Build history of the part. All positions in model axes, mm. A direction names the side the tool comes from. Round coordinates to 2 decimals unless told otherwise and drop trailing zeros. Order: outer loops, then holes, each group sorted by start corner. A loop starts at its lowest first (then second) coordinate and runs counter-clockwise, first axis right, second up. Notation, with made-up numbers: (61, 52) - (91, 52) arc R20 cw to (91, 60) - close; hole circle Ø10 at (16.25, -35.75). An arc over 180 degrees is marked (long way). Write each question's results on one line, items separated by ' | '. Start each with the question number.
```python
from build123d import *

# Parameters (mm, degrees)
F1_DEPTH    = 41
F2_R        = 4
F3_T1_DEPTH = 51


# Not quite as in the source:
# - a fillet or chamfer that OpenCascade refuses, or shapes differently, is made with other operations: its cross-section is extruded or revolved along the edge and cut away or added


with BuildPart() as f1:
    # F0 (on Front) → F1 (new body)
    with BuildSketch(Plane.XZ):
        Polygon((-42.5, 18.5), (-39, 18.5), (-39, 38.5), (-17.5, 38.5), (-17.5, 21.5), (-3.5, 21.5), (-3.5, -3.5), (0, -3.5), (0, 0), (0, 25), (-14, 25), (-14, 42), (-42.5, 42), align=None)
        Polygon((0, 0), (0, -3.5), (33.5, -3.5), (33.5, -147.2), (13.5, -147.2), (13.5, -150.7), (37, -150.7), (37, 0), align=None)
    extrude(amount=F1_DEPTH)

    # F2
    f2_edges = [f1.edges().sort_by_distance(p)[0] for p in [
        (-42.5, -20.5, 42),
        (-14, -20.5, 42),
        (0, -20.5, 25),
        (0, -20.5, 0),
        (-14, -20.5, 25),
        (37, -20.5, 0),
        (37, -20.5, -150.7),
        (-3.5, -20.5, -3.5),
    ]]
    fillet(f2_edges, radius=F2_R)

    # F3: fillet of radius 2 on 4 edges, made by hand

    # F3_s2 → F3_t1 (cut)
    with BuildSketch(Plane.XZ.offset(-5)):
        with BuildLine():
            ThreePointArc((-40.5, 18.5), (-41.9142135624, 19.0857864376), (-42.5, 20.5))
            Line((-42.5, 20.5), (-42.5, 18.5))
            Line((-42.5, 18.5), (-40.5, 18.5))
        make_face()
        with BuildLine():
            ThreePointArc((15.5, -147.2), (14.0857864376, -147.7857864376), (13.5, -149.2))
            Line((13.5, -149.2), (13.5, -147.2))
            Line((13.5, -147.2), (15.5, -147.2))
        make_face()
        with BuildLine():
            ThreePointArc((13.5, -148.7), (14.0857864376, -150.1142135624), (15.5, -150.7))
            Line((15.5, -150.7), (13.5, -150.7))
            Line((13.5, -150.7), (13.5, -148.7))
        make_face()
        with BuildLine():
            ThreePointArc((-15.5, 21.5), (-16.9142135624, 22.0857864376), (-17.5, 23.5))
            Line((-17.5, 23.5), (-17.5, 21.5))
            Line((-17.5, 21.5), (-15.5, 21.5))
        make_face()
    extrude(amount=F3_T1_DEPTH, mode=Mode.SUBTRACT)


solid = f1.part
```
1. Cut at D-D (x = -8). List the corners of the cut face in (y, z), plus the area to 4 significant figures.
2. 3-axis set-ups, long thin cutter, end or side, ignore diameter. For faces 5 (the face through (0, -20, 12)), 6 (the face through (17, -20, -3.5)), 7 (the face through (-42.5, -20, 29)): which of +Z, -Z, +X, -X, +Y, -Y reach the whole face in a straight line?
3. Cut at C-C (z = -129). List the corners of the cut face in (x, y).
4. Cut at B-B (x = 19.5). List the corners of the cut face in (y, z).
5. Wall check: line 1 (X direction, y = -13, z = 34); line 2 (Z direction, x = 25, y = -9.5); line 3 (Z direction, x = -8.5, y = -23.5). Give the ranges that are in metal, low to high. Write a range as from..to.
6. Flat gauge pins, fed straight in: pin 1 Ø1.5 at (y, z) = (-11.5, -0.5) entering from +X; pin 2 Ø6.5 at (x, y) = (-8, -24.5) entering from +Z; pin 3 Ø11 at (x, y) = (-28, -15.5) entering from -Z; pin 4 Ø23 at (y, z) = (-27, 10) entering from -X. Where does each tip first touch, or does it go through?
7. Mould opens along Z. For faces 1 (the face through (-3, -41, 3)), 2 (the face through (25, -20, -147.2)), 3 (the face through (-7, -20, 25)), 4 (the face through (-2.359, -20.787, -2.297)) say: pulls with the +Z half, pulls with the -Z half, needs draft (parallel to the pull), parting line crosses it, or undercut.
A:
1) outline: (-41, 21.5) - (0, 21.5) - (0, 25) - (-41, 25) - close | area: 143.5 mm^2
2) face 5: +Z, +X, +Y, -Y | face 6: -X, +Y, -Y | face 7: +Z, -Z, -X, +Y, -Y
3) outline: (33.5, -41) - (37, -41) - (37, 0) - (33.5, 0) - close
4) outline: (-41, -150.7) - (0, -150.7) - (0, -147.2) - (-41, -147.2) - close; (-41, -3.5) - (0, -3.5) - (0, 0) - (-41, 0) - close
5) line 1: x = -42.5..-39, -17.5..-14 | line 2: z = -150.7..-147.2, -3.5..0 | line 3: z = 21.5..25
6) pin 1: stops at x = 35.9 | pin 2: stops at z = 25.2 | pin 3: stops at z = 38.5 | pin 4: stops at x = -42.5
7) face 1: needs draft | face 2: undercut | face 3: pulls with the +Z half | face 4: pulls with the -Z half
